Can you work these out from the model? Positions are in its coordinate system, mm. A direction names the side the tool comes from. Coordinates: 2 decimals unless noted, no trailing zeros. Order: outer loops, then holes, each group sorted by start corner. A loop starts at its lowest first (then second) coordinate and runs counter-clockwise, first axis right, second up. Notation, with made-up numbers: (23.25, -5.5) -> (80.25, -5.5) arc R12 cw to (80.25, 6.5) -> close; hole circle Ø5 at (83, 1.5). An arc over 180 degrees is marked (long way). Use a Markdown table: item, result. Add a question column.
1. If I drill on line 1 along X through (y, z) = (14, 4.5); line 2 along X through (y, z) = (30, -1); line 3 along Z through (x, y) = (-14, 16), over which ranges is the centre line in solid material (lowest first)? Write a range as from..to.
2. For pin 1 Ø2.5 at (y, z) = (22.5, -6) entering from -X; pin 2 Ø18 at (y, z) = (50, -5) entering from -X; pin 3 Ø3 at (x, y) = (19.5, 33.5) entering from +Z, each with a flat end and sliding along its axis, tell me the tip position at first contact or that it passes through.
3. For faces 5 (the flat face through (7, 35, 2.4)), 6 (the flat face through (0, 35, -19.102)), 7 (the flat face through (-6, 35, -10.1)), which set-ups out of +Z, -Z, +X, -X, +Y, -Y let a thin tool reach every point of the face, with its end or its side?
4. Suppose I cut it at B-B, the plane x = 6. List the corners of the cut face in (y, z) for me.
5. Suppose I cut it at C-C, the plane y = 16.5. List the corners of the cut face in (x, z) for me.
6. Suppose I cut it at A-A, the plane z = -6. List the corners of the cut face in (x, y) for me.
7. Suppose I cut it at D-D, the plane z = -28.5. List the corners of the cut face in (x, y) for me, then the cut area to 3 significant figures.
8. We'd pull the mould along X, two halves only. Please class faces 1 (the flat face through (-25.17, 34.51, -31.84)), 2 (the flat face through (14.35, 34.51, -26.21)), 3 (the flat face through (20.601, 34.51, -20.178)), 4 (the flat face through (-7, 35, -2.4)): pulls with the +X half, pulls with the -X half, needs draft (parallel to the pull), parting line crosses it, or undercut.
```python
from build123d import *

# Parameters (mm, degrees)
BOSS_EXTRU_2_DEPTH = 70


with BuildPart() as part:
    # Base → Boss.-Extru.2 (new body)
    with BuildSketch(Plane(origin=(0, 0, 0), x_dir=(1, 0, 0), z_dir=(0, 1, 0))):
        Polygon((-3.85, -2.4), (-3.85, 2.4), (-10.1, 2.4), (-10.1, 10.1), (-2.4, 10.1), (-2.4, 3.85), (2.4, 3.85), (2.4, 10.1), (10.1, 10.1), (10.1, 2.4), (3.85, 2.4), (3.85, -2.4), (10.1, -2.4), (10.1, -6.247725424), (15.4, -6.247725424), (15.4, 10.102274576), (25.950506613, 30.539662134), (24.407491309, 33.11242403), (4, 19.102274576), (-4, 19.102274576), (-24.407491309, 33.11242403), (-25.950506613, 30.539662134), (-15.4, 10.102274576), (-15.4, -6.247725424), (-10.1, -6.247725424), (-10.1, -2.4), align=None)
    extrude(amount=BOSS_EXTRU_2_DEPTH)


solid = part.part
```
Worked out:
| question | item | result |
|---|---|---|
| 1 | line 1 | x = -15.4..-10.1, 10.1..15.4 |
| 1 | line 2 | x = -15.4..-3.85, 3.85..15.4 |
| 1 | line 3 | z = -25.97..6.25 |
| 2 | pin 1 | stops at x = -15.4 |
| 2 | pin 2 | stops at x = -17.41 |
| 2 | pin 3 | stops at z = -15.14 |
| 3 | face 5 | +Z, +Y, -Y |
| 3 | face 6 | -Z, +Y, -Y |
| 3 | face 7 | +Y, -Y |
| 4 | outline | (0, -20.48) -> (70, -20.48) -> (70, -10.1) -> (0, -10.1) -> close; (0, -2.4) -> (70, -2.4) -> (70, 2.4) -> (0, 2.4) -> close |
| 5 | outline | (-25.95, -30.54) -> (-24.41, -33.11) -> (-4, -19.1) -> (4, -19.1) -> (24.41, -33.11) -> (25.95, -30.54) -> (15.4, -10.1) -> (15.4, 6.25) -> (10.1, 6.25) -> (10.1, 2.4) -> (3.85, 2.4) -> (3.85, -2.4) -> (10.1, -2.4) -> (10.1, -10.1) -> (2.4, -10.1) -> (2.4, -3.85) -> (-2.4, -3.85) -> (-2.4, -10.1) -> (-10.1, -10.1) -> (-10.1, -2.4) -> (-3.85, -2.4) -> (-3.85, 2.4) -> (-10.1, 2.4) -> (-10.1, 6.25) -> (-15.4, 6.25) -> (-15.4, -10.1) -> close |
| 6 | outline | (-15.4, 0) -> (-10.1, 0) -> (-10.1, 70) -> (-15.4, 70) -> close; (-2.4, 0) -> (2.4, 0) -> (2.4, 70) -> (-2.4, 70) -> close; (10.1, 0) -> (15.4, 0) -> (15.4, 70) -> (10.1, 70) -> close |
| 7 | outline | (-24.9, 0) -> (-17.69, 0) -> (-17.69, 70) -> (-24.9, 70) -> close; (17.69, 0) -> (24.9, 0) -> (24.9, 70) -> (17.69, 70) -> close |
| 7 | area | 1,010 mm² |
| 8 | face 1 | pulls with the -X half |
| 8 | face 2 | undercut |
| 8 | face 3 | pulls with the +X half |
| 8 | face 4 | undercut |
